Build history of the part. All positions in model axes, mm. Face numbers are marked on the shaded views. A direction names the side the tool comes from. Coordinates: 2 decimals unless noted, no trailing zeros. Loops run counter-clockwise (first coordinate to the right, second up) from the corner with the lowest first, then second, coordinate; pieces in that order, holes last.
Item 1: Cut at D-D (z = -10). List the corners of the cut face in (x, y), and give its area (3 significant figures).
Item 2: Mould opens along X. For the marked faces 3, 4 and 5 say: released by +X, released by -X, zero draft, split by the parting line, or undercut.
Item 3: Cut at C-C (x = -5). List the corners of the cut face in (y, z), and give its area (3 significant figures).
Item 4: Cut at B-B (x = -22). List the corners of the cut face in (y, z), and give its area (3 significant figures).
Item 5: Flat gauge pins, fed straight in: pin 1 (3 mm diameter, centred on y = 2, z = -10.5, fed in from +X); pin 2 (3 mm diameter, centred on y = 1.5, z = -33.5, fed in from -X). Where does each tip first touch, or does it go through?
Item 6: Drill centre lines: line 1 along Z through (x, y) = (-5, 3.3); line 2 along X through (y, z) = (1.4, -30); line 3 along X through (y, z) = (0.5, -13). Where is each one in solid material? Low to high.
Item 7: 3-axis set-ups, long thin cutter, end or side, ignore diameter. For the marked faces 1 and 2: which of +Z, -Z, +X, -X, +Y, -Y reach the whole face in a straight line?
Item 8: Cut at A-A (z = -5.5). List the corners of the cut face in (x, y), and give its area (3 significant figures).
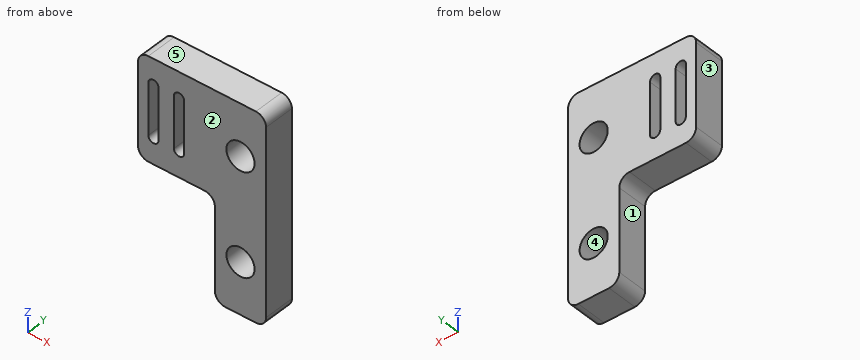
Autodesk Inventor part; units mm, degrees
ref_plane "YZ Plane" through (0, 0, 0) normal (1, 0, 0) x (0, 1, 0)
ref_plane "XZ Plane" through (0, 0, 0) normal (0, 1, 0) x (-1, 0, 0)
ref_plane "XY Plane" through (0, 0, 0) normal (0, 0, 1) x (1, 0, 0)
sketch "Sketch1" plane through (0, 0, 0) normal (0, 1, 0) x (-1, 0, 0)
  line L0 (0, 0) -> (10, 0)
  line L1 (10, 0) -> (10, -40)
  line L2 (10, -40) -> (0, -40)
  line L3 (0, -40) -> (0, 0)
  line L4 (10, 0) -> (25, 0)
  line L5 (25, 0) -> (25, -20)
  line L6 (25, -20) -> (10, -20)
  line L7 (10, -20) -> (10, 0)
  dimension "d0" = 10
  dimension "d1" = 40
  dimension "d2" = 15
  dimension "d3" = 20
extrude "Extrusion1" add sketch "Sketch1" along normal blind 6
sketch "Sketch2" plane through (0, 6, 0) normal (0, 1, 0) x (1, 0, 0)
  circle A0 centre (-5, 10) radius 2.75
  line L0 (0, 0) -> (0, 40)
  line L1 (-25, 0) -> (0, 0)
  circle A1 centre (-5, 30) radius 2.75
  line L2 (-25, 20) -> (-25, 0)
  line L3 (-25, 10) -> (-22, 10)
  line L4 (-22, 10) -> (-17, 10)
  line L5 (-22, 5) -> (-22, 15) construction
  line L6 (-21, 5) -> (-21, 15)
  line L7 (-23, 15) -> (-23, 5)
  arc A2 (-23, 5) -> (-21, 5) centre (-22, 5) ccw
  arc A3 (-21, 15) -> (-23, 15) centre (-22, 15) ccw
  line L8 (-17, 5) -> (-17, 15) construction
  line L9 (-16, 5) -> (-16, 15)
  line L10 (-18, 15) -> (-18, 5)
  arc A4 (-18, 5) -> (-16, 5) centre (-17, 5) ccw
  arc A5 (-16, 15) -> (-18, 15) centre (-17, 15) ccw
  line L11 (-17, 10) -> (-7, 10) construction
  dimension "d6" = 5.5
  dimension "d7" = 5
  dimension "d8" = 10
  dimension "d9" = 5.5
  dimension "d10" = 5
  dimension "d11" = 20
  dimension "d12" = 3
  dimension "d13" = 5
  dimension "d14" = 5
  dimension "d15" = 2
  dimension "d16" = 5
  dimension "d17" = 90
  dimension "d18" = 2
extrude "Extrusion2" cut sketch "Sketch2" against normal up to next
fillet "Fillet1" radius 2 6 edges at (0, 3, 0) (-25, 3, 0) (0, 3, -40) (-10, 3, -40) (-10, 3, -20) (-25, 3, -20)
properties part number "Small_Belt_Clamp"
Filled sheet:
1. outline: (-25, 0) - (-23, 0) - (-23, 6) - (-25, 6) - close; (-21, 0) - (-18, 0) - (-18, 6) - (-21, 6) - close; (-16, 0) - (-7.75, 0) - (-7.75, 6) - (-16, 6) - close; (-2.25, 0) - (0, 0) - (0, 6) - (-2.25, 6) - close
1. area: 93.0 mm2
2. face 3: released by -X
2. face 4: undercut
2. face 5: zero draft
3. outline: (0, -40) - (6, -40) - (6, -32.75) - (0, -32.75) - close; (0, -27.25) - (6, -27.25) - (6, -12.75) - (0, -12.75) - close; (0, -7.25) - (6, -7.25) - (6, 0) - (0, 0) - close
3. area: 174 mm2
4. outline: (0, -20) - (6, -20) - (6, -16) - (0, -16) - close; (0, -4) - (6, -4) - (6, 0) - (0, 0) - close
4. area: 48.0 mm2
5. pin 1: stops at x = 0
5. pin 2: stops at x = -10
6. line 1: z = -40 to -32.75, -27.25 to -12.75, -7.25 to 0
6. line 2: x = -10 to -7.75, -2.25 to 0
6. line 3: x = -25 to -23, -21 to -18, -16 to 0
7. face 1: -Z, -X, +Y, -Y
7. face 2: +Z, -Z, +X, -X, -Y
8. outline: (-25, 0) - (-23, 0) - (-23, 6) - (-25, 6) - close; (-21, 0) - (-18, 0) - (-18, 6) - (-21, 6) - close; (-16, 0) - (0, 0) - (0, 6) - (-16, 6) - close
8. area: 126 mm2
